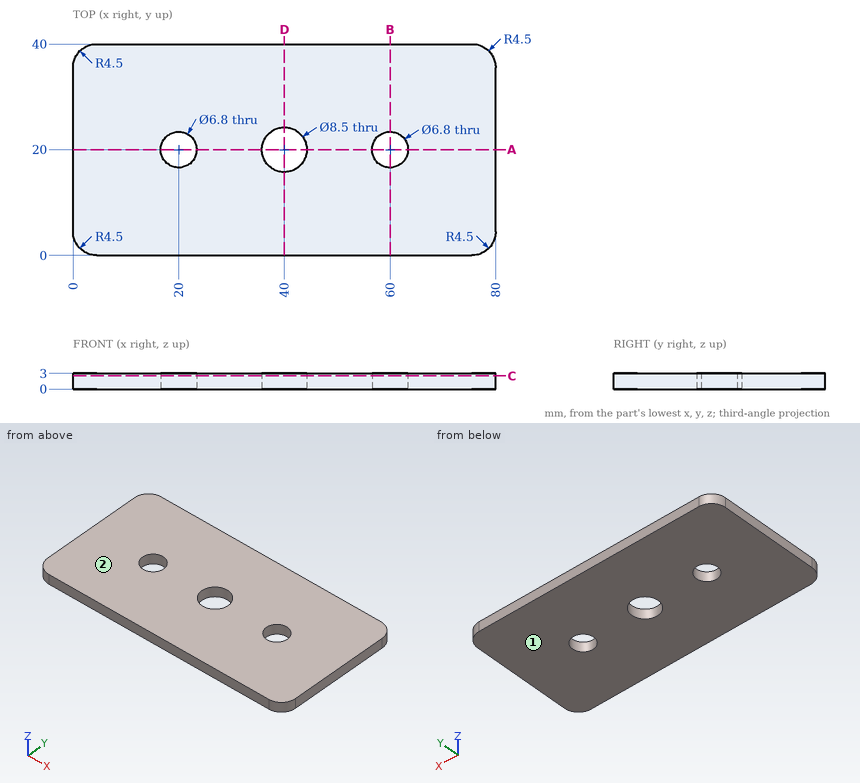
Could you check a few things on this drawing? It's one solid part, dimensions in mm from its lowest x, y, z. Round coordinates to 2 decimals unless told otherwise and drop trailing zeros. Write each loop counter-clockwise with the first axis right and the second up, starting at its lowest first coordinate (ties: lowest second). Pieces come first, ordered by that corner, then holes.
Q1. If we section it at B-B on x = 60: Write out the boundary of the cut face in (y, z), plus the area to 3 significant figures.
Q2. If we section it at A-A on y = 20: Write out the boundary of the cut face in (x, z), plus the area to 3 significant figures.
Q3. If we section it at C-C on z = 2.5: Write out the boundary of the cut face in (x, y), plus the area to 3 significant figures.
Q4. If we section it at D-D on x = 40: Write out the boundary of the cut face in (y, z).
Q5. Please list where these lines run through material, in increasing order: probe 1 along Y at (x, z) = (60, 1.9); probe 2 along X at (y, z) = (22, 1.5); probe 3 along Y at (x, z) = (40, 0.65).
Q6. Will these pins go through, and if not, where does the flat tip stop? P1, Ø1.5, axis at x = 38, y = 17, coming from the +Z side; P2, Ø4, axis at x = 60, y = 20, coming from the -Z side.
Q7. If we mould it in two halves opening along Z, with no side actions, what happens to the marked faces 1 and 2? For each: +Z half, -Z half, draft (parallel to the pull), parting line (faces both ways), or undercut.
Answer below:
1. outline: (0, 0) - (16.6, 0) - (16.6, 3) - (0, 3) - close; (23.4, 0) - (40, 0) - (40, 3) - (23.4, 3) - close
1. area: 99.6 mm2
2. outline: (0, 0) - (16.6, 0) - (16.6, 3) - (0, 3) - close; (23.4, 0) - (35.75, 0) - (35.75, 3) - (23.4, 3) - close; (44.25, 0) - (56.6, 0) - (56.6, 3) - (44.25, 3) - close; (63.4, 0) - (80, 0) - (80, 3) - (63.4, 3) - close
2. area: 174 mm2
3. outline: (0, 4.5) arc R4.5 ccw to (4.5, 0) - (75.5, 0) arc R4.5 ccw to (80, 4.5) - (80, 35.5) arc R4.5 ccw to (75.5, 40) - (4.5, 40) arc R4.5 ccw to (0, 35.5) - close; hole circle Ø6.8 at (20, 20); hole circle Ø8.5 at (40, 20); hole circle Ø6.8 at (60, 20)
3. area: 3,050 mm2
4. outline: (0, 0) - (15.75, 0) - (15.75, 3) - (0, 3) - close; (24.25, 0) - (40, 0) - (40, 3) - (24.25, 3) - close
5. probe 1: y = 0 to 16.6, 23.4 to 40
5. probe 2: x = 0 to 17.25, 22.75 to 36.25, 43.75 to 57.25, 62.75 to 80
5. probe 3: y = 0 to 15.75, 24.25 to 40
6. P1: stops at z = 3
6. P2: passes through
7. face 1: -Z half
7. face 2: +Z half
